CAD build for the part. Positions are in the model's coordinates, mm. Face numbers are marked on the shaded views. A direction names the side the tool comes from. Give positions to 0.01 mm unless a question says otherwise; leave off trailing zeros. Loops run counter-clockwise (first coordinate to the right, second up) from the corner with the lowest first, then second, coordinate; pieces in that order, holes last.
Item 1: Saw through at C-C on x = -18. Give the cut face in (y, z).
Item 2: Which spindle directions (+Z, -Z, +X, -X, +Y, -Y) get a long thin tool onto all of the face, cutting with end or side? Do the marked faces 4, 5, 6 and 7. Say none if no direction does.
Item 3: Saw through at B-B on z = 10.75. Give the cut face in (x, y), plus the area to 3 significant figures.
Item 4: Saw through at D-D on z = 15.75. Give the cut face in (x, y) (3 decimals).
Item 5: Probe probe 1 along X at (y, z) = (-4.55, 17.5) (3 decimals); probe 2 along Y at (x, z) = (1.65, 15.85) (3 decimals); probe 3 along Y at (x, z) = (-9, 3.5). List the from-to ranges inside material, lowest first.
Item 6: Mould opens along X. For the marked faces 1, 2 and 3 say: released by +X, released by -X, zero draft, split by the parting line, or undercut.
Item 7: Saw through at A-A on y = -7.75. Give the cut face in (x, z), plus the area to 3 significant figures.
Item 8: Drop flat-ended pins along their axis: P1, Ø5, axis at y = 0.5, z = 6, coming from the +X side; P2, Ø2.5, axis at x = 1.65, y = -4.55, coming from the -Z side; P3, Ø2, axis at x = -27, z = 15.5, coming from the -Y side; P4, Ø5, axis at y = -3.5, z = 11.5, coming from the +X side. Give the stop position or say it passes through.
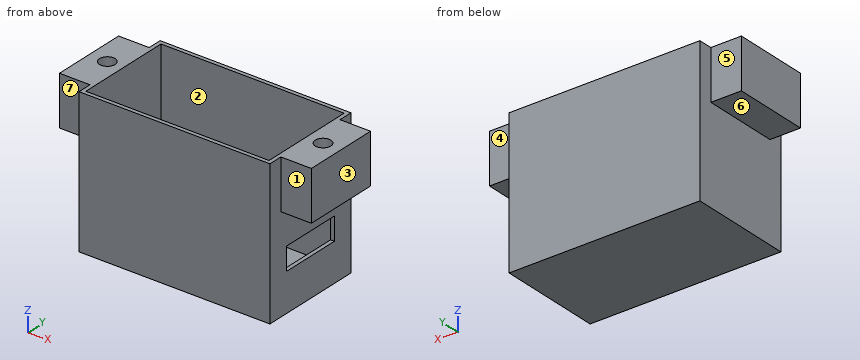
Autodesk Fusion 360 part; units mm, degrees
sketch "Sketch1" plane through (0, 0, 0) normal (0, 0, 1) x (1, 0, 0)
  line L0 (-25, -11.4) -> (-25, 2.3)
  line L1 (-25, 2.3) -> (0, 2.3)
  line L2 (0, 2.3) -> (0, -11.4)
  line L3 (0, -11.4) -> (-25, -11.4)
  dimension "d1" = 13.7
  dimension "d2" = 25
extrude "Extrude1" add sketch "Sketch1" along normal blind 19
shell "Shell1" thickness 0.5 removed faces 1 at (-8.3333, -6.8333, 19)
sketch "Sketch2" plane through (0, 0, 0) normal (1, 0, 0) x (0, 1, 0)
  line L0 (-11.4, 0) -> (2.3, 0)
  line L1 (2.3, 0) -> (2.3, 19)
  line L2 (2.3, 19) -> (-11.4, 19)
  line L3 (-11.4, 19) -> (-11.4, 0)
  line L4 (-8.6, 8) -> (-0.5, 8)
  line L5 (-0.5, 8) -> (-0.5, 5)
  line L6 (-0.5, 5) -> (-8.6, 5)
  line L7 (-8.6, 5) -> (-8.6, 8)
  dimension "d6" = 5
  dimension "d7" = 8.1
  dimension "d8" = 2.8
  dimension "d9" = 2.8
extrude "Extrude2" cut sketch "Sketch2" along normal mid plane 6 contours L4 L5 L6 L7
sketch "Sketch3" plane through (0, 0, 0) normal (1, 0, 0) x (0, 1, 0)
  line L0 (-0.5, 8) -> (-0.5, 5)
  line L1 (-0.5, 5) -> (-8.6, 5)
  line L2 (-8.6, 5) -> (-8.6, 8)
  line L3 (-8.6, 8) -> (-0.5, 8)
  line L4 (-11.4, 0) -> (2.3, 0)
  line L5 (2.3, 0) -> (2.3, 19)
  line L6 (2.3, 19) -> (-11.4, 19)
  line L7 (-11.4, 19) -> (-11.4, 0)
  line L8 (-9.55, 19) -> (0.45, 19)
  line L9 (0.45, 19) -> (0.45, 12.5)
  line L10 (0.45, 12.5) -> (-9.55, 12.5)
  line L11 (-9.55, 12.5) -> (-9.55, 19)
  dimension "d19" = 10
  dimension "d20" = 1.85
  dimension "d23" = 6.5
extrude "Extrude3" add sketch "Sketch3" along normal blind 4 contours L6 L8 L9 L10 L11
sketch "Sketch4" plane through (0, 0, 19) normal (0, 0, 1) x (-1, 0, 0)
  line L0 (0.5, 10.9) -> (24.5, 10.9)
  line L1 (24.5, 10.9) -> (24.5, -1.8)
  line L2 (24.5, -1.8) -> (0.5, -1.8)
  line L3 (0.5, -1.8) -> (0.5, 10.9)
  line L4 (0, 11.4) -> (0, 9.55)
  line L5 (0, 9.55) -> (-4, 9.55)
  line L6 (-4, 9.55) -> (-4, -0.45)
  line L7 (-4, -0.45) -> (0, -0.45)
  line L8 (0, -0.45) -> (0, -2.3)
  line L9 (0, -2.3) -> (25, -2.3)
  line L10 (25, -2.3) -> (25, 11.4)
  line L11 (25, 11.4) -> (0, 11.4)
  circle A0 centre (-1.65, 4.55) radius 1.025
  dimension "d16" = 2.05
  dimension "d32" = 5
  dimension "d33" = 2.15
extrude "Extrude4" cut sketch "Sketch4" against normal blind 5.5 contours A0
sketch "Sketch6" plane through (-25, 0, 0) normal (-1, 0, 0) x (0, -1, 0)
  line L0 (-2.3, 0) -> (11.4, 0)
  line L1 (11.4, 0) -> (11.4, 19)
  line L2 (11.4, 19) -> (-2.3, 19)
  line L3 (-2.3, 19) -> (-2.3, 0)
  line L4 (-0.45, 19) -> (9.55, 19)
  line L5 (9.55, 19) -> (9.55, 12.5)
  line L6 (9.55, 12.5) -> (-0.45, 12.5)
  line L7 (-0.45, 12.5) -> (-0.45, 19)
  dimension "d27" = 1.85
  dimension "d28" = 10
  dimension "d29" = 6.5
extrude "Extrude5" add sketch "Sketch6" along normal blind 4 contours L2 L4 L5 L6 L7
sketch "Sketch7" plane through (0, 0, 19) normal (0, 0, 1) x (-1, 0, 0)
  circle A0 centre (-1.65, 4.55) radius 1.025
  line L0 (0.5, 10.9) -> (24.5, 10.9)
  line L1 (24.5, 10.9) -> (24.5, -1.8)
  line L2 (24.5, -1.8) -> (0.5, -1.8)
  line L3 (0.5, -1.8) -> (0.5, 10.9)
  line L4 (0, 11.4) -> (0, 9.55)
  line L5 (0, 9.55) -> (-4, 9.55)
  line L6 (-4, 9.55) -> (-4, -0.45)
  line L7 (-4, -0.45) -> (0, -0.45)
  line L8 (0, -0.45) -> (0, -2.3)
  line L9 (0, -2.3) -> (25, -2.3)
  line L10 (25, -2.3) -> (25, -0.45)
  line L11 (25, -0.45) -> (29, -0.45)
  line L12 (29, -0.45) -> (29, 9.55)
  line L13 (29, 9.55) -> (25, 9.55)
  line L14 (25, 9.55) -> (25, 11.4)
  line L15 (25, 11.4) -> (0, 11.4)
  circle A1 centre (26.6, 4.55) radius 1.025
  dimension "d34" = 2.05
  dimension "d35" = 2.1
  dimension "d36" = 5
extrude "Extrude6" cut sketch "Sketch7" against normal blind 5.5 contours A1
Results below:
1. outline: (-11.4, 0) - (2.3, 0) - (2.3, 19) - (1.8, 19) - (1.8, 0.5) - (-10.9, 0.5) - (-10.9, 19) - (-11.4, 19) - close
2. face 4: +Z, -Z, +X, +Y
2. face 5: +Z, -Z, -X, +Y
2. face 6: -Z, -X, +Y, -Y
2. face 7: +Z, -Z, -X, -Y
3. outline: (-25, -11.4) - (0, -11.4) - (0, 2.3) - (-25, 2.3) - close; hole (-24.5, -10.9) - (-0.5, -10.9) - (-0.5, 1.8) - (-24.5, 1.8) - close
3. area: 37.7 mm2
4. outline: (-29, -9.55) - (-25, -9.55) - (-25, -11.4) - (0, -11.4) - (0, -9.55) - (4, -9.55) - (4, 0.45) - (0, 0.45) - (0, 2.3) - (-25, 2.3) - (-25, 0.45) - (-29, 0.45) - close; hole circle Ø2.05 at (-26.6, -4.55); hole (-24.5, -10.9) - (-0.5, -10.9) - (-0.5, 1.8) - (-24.5, 1.8) - close; hole circle Ø2.05 at (1.65, -4.55)
5. probe 1: x = -29 to -27.625, -25.575 to -24.5, -0.5 to 0.625, 2.675 to 4
5. probe 2: y = -9.55 to -5.575, -3.525 to 0.45
5. probe 3: y = -11.4 to -10.9, 1.8 to 2.3
6. face 1: zero draft
6. face 2: undercut
6. face 3: released by +X
7. outline: (-29, 12.5) - (-25, 12.5) - (-25, 0) - (0, 0) - (0, 5) - (-0.5, 5) - (-0.5, 0.5) - (-24.5, 0.5) - (-24.5, 19) - (-29, 19) - close; (-0.5, 8) - (0, 8) - (0, 12.5) - (4, 12.5) - (4, 19) - (-0.5, 19) - close
7. area: 81.5 mm2
8. P1: stops at x = 0
8. P2: stops at z = 12.5
8. P3: stops at y = -9.55
8. P4: stops at x = 4
